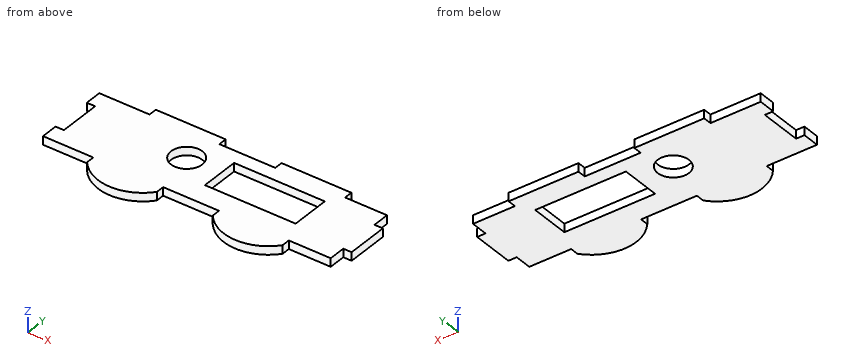
```python
from build123d import *

# Parameters (mm, degrees)
SKETCH_R      = 5.6
SKETCH_W      = 32.48
SKETCH_H      = 14
EXTRUDE_DEPTH = 3


with BuildPart() as part:
    # Sketch → Extrude (new body)
    with BuildSketch(Plane.XY):
        with BuildLine():
            Line((40, -6.37), (40, -9.37))
            ThreePointArc((15, -9.37), (27.5, -15.37), (40, -9.37))
            Line((15, -9.37), (15, -6.37))
            Line((15, -6.37), (0, -6.37))
            Line((-3, -6.37), (0, -6.37))
            Line((-3, -0.34), (-3, -6.37))
            Line((-3, -0.34), (0, -0.34))
            Line((0, 14.66), (0, -0.34))
            Line((0, 14.66), (-3, 14.66))
            Line((-3, 14.66), (-3, 20.66))
            Line((-3, 20.66), (0, 20.66))
            Line((0, 20.66), (15, 20.66))
            Line((15, 23.66), (15, 20.66))
            Line((40, 23.66), (15, 23.66))
            Line((40, 20.66), (40, 23.66))
            Line((40, 20.66), (60, 20.66))
            Line((60, 23.66), (60, 20.66))
            Line((85, 23.66), (60, 23.66))
            Line((85, 20.66), (85, 23.66))
            Line((85, 20.66), (100, 20.66))
            Line((100, 20.66), (100, 14.66))
            Line((100, 14.66), (103, 14.66))
            Line((103, 14.66), (103, -0.34))
            Line((103, -0.34), (100, -0.34))
            Line((100, -0.34), (100, -6.37))
            Line((100, -6.37), (85, -6.37))
            Line((85, -6.37), (85, -9.37))
            ThreePointArc((60, -9.37), (72.5, -15.37), (85, -9.37))
            Line((60, -9.37), (60, -6.37))
            Line((60, -6.37), (40, -6.37))
        make_face()
        with Locations((36.6, 9.5)):
            Circle(SKETCH_R, mode=Mode.SUBTRACT)
        with Locations((65.265, 8.6)):
            Rectangle(SKETCH_W, SKETCH_H, mode=Mode.SUBTRACT)
    extrude(amount=EXTRUDE_DEPTH)


solid = part.part
```
Input: part model. Units: mm. Frame: model coordinates. Coordinates: 2 decimals unless noted, no trailing zeros. Loops run counter-clockwise (first coordinate to the right, second up) from the corner with the lowest first, then second, coordinate; pieces in that order, holes last.
Q1. Section C-C, the plane x = 77. Return the cut outline in (y, z).
Results are:
outline: (-14.73, 0) - (1.6, 0) - (1.6, 3) - (-14.73, 3) - close; (15.6, 0) - (23.66, 0) - (23.66, 3) - (15.6, 3) - close
Q2. Section B-B, the plane y = 9.5. Return the cut outline in (x, z) (3 decimals), and give its area (3 significant figures).
Results are:
outline: (0, 0) - (31, 0) - (31, 3) - (0, 3) - close; (42.2, 0) - (49.025, 0) - (49.025, 3) - (42.2, 3) - close; (81.505, 0) - (103, 0) - (103, 3) - (81.505, 3) - close
area: 178 mm2
Q3. Section A-A, the plane y = -7.5. Return the cut outline in (x, z).
Results are:
outline: (15, 0) - (40, 0) - (40, 3) - (15, 3) - close; (60, 0) - (85, 0) - (85, 3) - (60, 3) - close
Q4. Line query: line 1 along X through (y, z) = (6.5, 1.5) (3 decimals); line 2 along X through (y, z) = (11.5, 0.95) (3 decimals); line 3 along Y through (x, z) = (3, 0.65). Output: solid intervals per line, ascending.
Results are:
line 1: x = 0 to 31.871, 41.329 to 49.025, 81.505 to 103
line 2: x = 0 to 31.369, 41.831 to 49.025, 81.505 to 103
line 3: y = -6.37 to 20.66
Q5. Contact query for flat-ended pins moving along their axis: pin 1 (0.9 mm diameter, centred on y = -8, z = 2, fed in from -X); pin 2 (0.9 mm diameter, centred on y = 22.5, z = 1.5, fed in from +X); pin 3 (0.9 mm diameter, centred on x = 92.5, z = 1.5, fed in from -Y). Output: stop coordinate, or through.
Results are:
pin 1: stops at x = 15
pin 2: stops at x = 85
pin 3: stops at y = -6.37
Q6. Section D-D, the plane z = 0.95. Give the number of separate pieces and of enclosed holes in the cut face, and give its area (3 significant figures).
Results are:
separate pieces: 1
enclosed holes: 2
area: 2,740 mm2
